Could you check a few things on this drawing? It's one solid part, dimensions in mm from its lowest x, y, z. Give positions to 0.01 mm unless a question says otherwise; leave off trailing zeros. Loops run counter-clockwise (first coordinate to the right, second up) from the corner with the lowest first, then second, coordinate; pieces in that order, holes last. Notation, with made-up numbers: (77, 39.25) -> (100, 39.25) arc R20 cw to (100, 52.25) -> close; hole circle Ø5 at (27.25, 67.25). An arc over 180 degrees is marked (long way). Use CSV: the item, a comma, the result in double quotes.
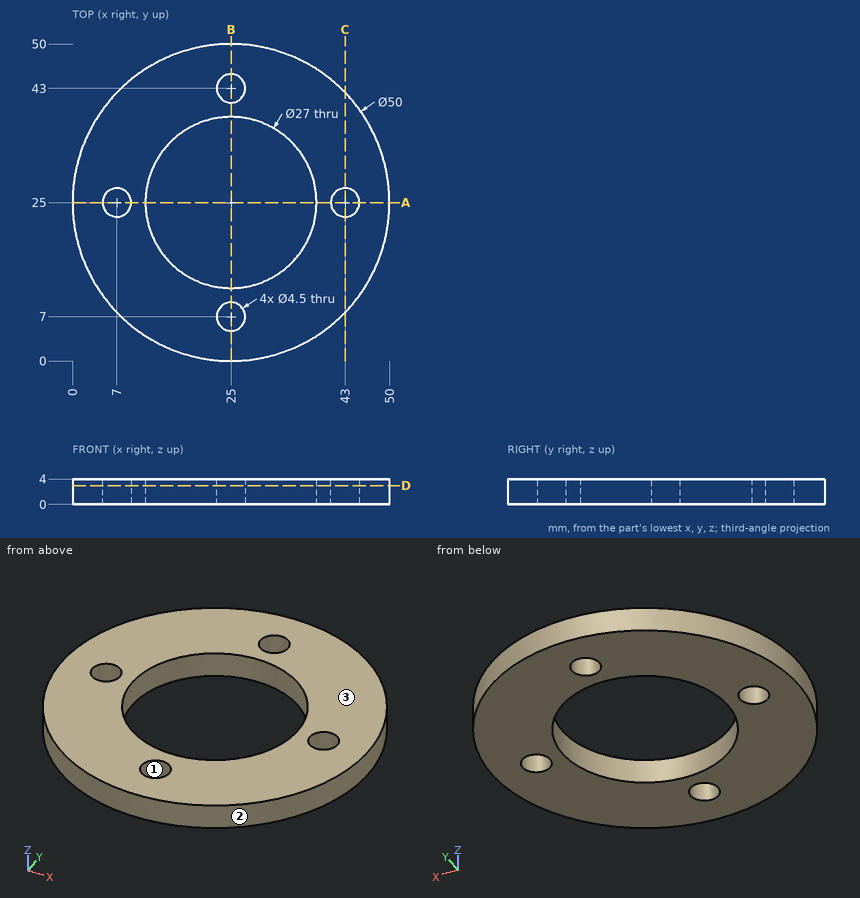
(1) If I drill on L1, parallel to Y at x = 26, z = 1.35; L2, parallel to Y at x = 6, z = 2.75; L3, parallel to Y at x = 8.5, z = 3.8, over which ranges is the centre line in solid material (lowest first)? Write a range as from..to.
Answer sheet:
L1,"y = 0.02..4.98, 9.02..11.54, 38.46..40.98, 45.02..49.98"
L2,"y = 8.75..22.98, 27.02..41.25"
L3,"y = 6.22..23.32, 26.68..43.78"
(2) If we section it at C-C, the plane x = 43: Write out the boundary of the cut face in (y, z).
Answer sheet:
outline,"(7.65, 0) -> (22.75, 0) -> (22.75, 4) -> (7.65, 4) -> close; (27.25, 0) -> (42.35, 0) -> (42.35, 4) -> (27.25, 4) -> close"
(3) Will this pin go through, and if not, where does the flat tip stop? pin 1 Ø21.5 at (x, y) = (25, 25) entering from -Z.
Answer sheet:
pin 1,"passes through"
(4) We'd pull the mould along Y, two halves only. Please class the marked faces 1, 2 and 3: released by +Y, released by -Y, zero draft, split by the parting line, or undercut.
Answer sheet:
face 1,"undercut"
face 2,"split by the parting line"
face 3,"zero draft"
(5) If we section it at A-A, the plane y = 25: Write out the boundary of the cut face in (x, z).
Answer sheet:
outline,"(0, 0) -> (4.75, 0) -> (4.75, 4) -> (0, 4) -> close; (9.25, 0) -> (11.5, 0) -> (11.5, 4) -> (9.25, 4) -> close; (38.5, 0) -> (40.75, 0) -> (40.75, 4) -> (38.5, 4) -> close; (45.25, 0) -> (50, 0) -> (50, 4) -> (45.25, 4) -> close"
(6) If we section it at D-D, the plane z = 2.95: Write out the boundary of the cut face in (x, y).
Answer sheet:
outline,"circle Ø50 at (25, 25); hole circle Ø4.5 at (7, 25); hole circle Ø27 at (25, 25); hole circle Ø4.5 at (25, 7); hole circle Ø4.5 at (25, 43); hole circle Ø4.5 at (43, 25)"
